```python
from build123d import *

# Parameters (mm, degrees)
SKETCH_1_R      = 2.899935842
EXTRUDE_1_DEPTH = 1


with BuildPart() as part:
    # 草圖1 → 填料-伸長1 (new body)
    with BuildSketch(Plane.XY):
        Circle(SKETCH_1_R)
        with BuildLine():
            ThreePointArc((0, 2.326630403), (-1.271608832, 1.94838908), (-2.129765657, 0.936646827))
            ThreePointArc((-2.129765657, 0.936646827), (-1.873360766, 0.277665392), (-1.21437933, 0.534070283))
            ThreePointArc((-1.21437933, 0.534070283), (-0.725063566, 1.110959518), (0, 1.326630403))
            ThreePointArc((0, 1.326630403), (0.5, 1.826630403), (0, 2.326630403))
        make_face(mode=Mode.SUBTRACT)
    extrude(amount=EXTRUDE_1_DEPTH)


solid = part.part
```
Verification items for the finished model (mm, model axes). A direction names the side the tool comes from. Round coordinates to 2 decimals unless told otherwise and drop trailing zeros. Write each loop counter-clockwise with the first axis right and the second up, starting at its lowest first coordinate (ties: lowest second). Pieces come first, ordered by that corner, then holes. Notation, with made-up numbers: (68, 25) -> (89, 25) arc R18 ccw to (89, 40) -> close; hole circle Ø4 at (37.5, 14). An arc over 180 degrees is marked (long way). Write each question's results on one line, items separated by ' | '.
Q1. Sectioned sample at A-A, the plane z = 0.85. Record the boundary of the cut face in (x, y).
Derived:
outline: circle Ø5.8 at (0, 0); hole (-2.13, 0.94) arc R0.5 ccw to (-1.21, 0.53) arc R1.33 cw to (0, 1.33) arc R0.5 ccw to (0, 2.33) arc R2.33 ccw to start
Q2. Sectioned sample at B-B, the plane y = 2.25. Record the boundary of the cut face in (x, z), and give its area (3 significant figures).
Derived:
outline: (-1.83, 0) -> (-0.59, 0) -> (-0.59, 1) -> (-1.83, 1) -> close; (0.27, 0) -> (1.83, 0) -> (1.83, 1) -> (0.27, 1) -> close | area: 2.80 mm²
Q3. Thickness scan on probe 1 along X at (y, z) = (1.85, 0.05); probe 2 along Y at (x, z) = (-0.5, 0.7); probe 3 along Y at (x, z) = (-1, 0.9). Record the ranges inside material, lowest first.
Derived:
probe 1: x = -2.23 to -1.41, 0.5 to 2.23 | probe 2: y = -2.86 to 1.23, 2.27 to 2.86 | probe 3: y = -2.72 to 0.87, 2.1 to 2.72
Q4. Sectioned sample at C-C, the plane x = -2.05. Record the boundary of the cut face in (y, z).
Derived:
outline: (-2.05, 0) -> (0.41, 0) -> (0.41, 1) -> (-2.05, 1) -> close; (1.1, 0) -> (2.05, 0) -> (2.05, 1) -> (1.1, 1) -> close
Q5. Draft check along Y on faces 3 (the face through (0, 0, 0)), 4 (the face through (0.5, 1.8, 0.5)), 5 (the face through (-0.378, 2.875, 0.493)). Enter one of: released by +Y, released by -Y, zero draft, split by the parting line, or undercut.
Derived:
face 3: zero draft | face 4: undercut | face 5: split by the parting line
Q6. Sectioned sample at D-D, the plane x = 1.2. Record the boundary of the cut face in (y, z), and give its area (3 significant figures).
Derived:
outline: (-2.64, 0) -> (2.64, 0) -> (2.64, 1) -> (-2.64, 1) -> close | area: 5.28 mm²
Q7. Access from +Z, -Z, +X, -X, +Y, -Y to the whole of each face (thin tool, end or side, straight path). Record for faces 1 (the face through (-1.256, 1.959, 0.493)), 2 (the face through (0, 0, 1)).
Derived:
face 1: +Z, -Z | face 2: +Z, +X, -X, +Y, -Y
